Autodesk Inventor part; units mm, degrees
ref_plane "YZ Plane" through (0, 0, 0) normal (1, 0, 0) x (0, 1, 0)
ref_plane "XZ Plane" through (0, 0, 0) normal (0, 1, 0) x (-1, 0, 0)
ref_plane "XY Plane" through (0, 0, 0) normal (0, 0, 1) x (1, 0, 0)
sketch "Sketch1" plane through (0, 0, 0) normal (0, 1, 0) x (-1, 0, 0)
  arc A0 (7, 0) -> (-7, 0) centre (0, 0) ccw
  circle A1 centre (0, 0) radius 4
  line L0 (-7, 0) -> (-7, -83)
  line L1 (-7, -83) -> (7, -83)
  line L2 (7, -83) -> (7, 0)
  point P0 (0, -83)
  dimension "d0" = 14
  dimension "d1" = 8
  dimension "d2" = 83
  dimension "d3" = 14
  dimension "d4" = 83
  dimension "d5" = 0
extrude "Extrusion1" add sketch "Sketch1" along normal blind 20
sketch "Sketch2" plane through (7, 0, 0) normal (1, 0, 0) x (0, 0, -1)
  line L0 (0, 20) -> (83, 20)
  line L1 (83, 0) -> (83, 20)
  line L2 (83, 20) -> (81.9518, 0)
  line L3 (83, 20) -> (107.3414, 20) construction
  line L4 (83, 20) -> (83, 0)
  line L5 (83, 0) -> (81.9518, 0)
  line L6 (0, 0) -> (83, 0)
  dimension "d9" = 93
extrude "Extrusion2" cut sketch "Sketch2" against normal through all
sketch "Sketch3" plane through (7, 0, 0) normal (1, 0, 0) x (0, 0, -1)
  line L0 (-7, 6) -> (8, 6)
  line L1 (8, 6) -> (8, 14)
  line L2 (8, 14) -> (-7, 14)
  line L3 (-7, 14) -> (-7, 6)
  line L4 (-7, 6) -> (8, 14) construction
  line L5 (8, 6) -> (-7, 14) construction
  point P0 (0, 0)
  point P1 (0.5, 10)
  dimension "d12" = 10
  dimension "d13" = 15
  dimension "d14" = 8
  dimension "d15" = 7
extrude "Extrusion3" cut sketch "Sketch3" against normal through all
chamfer "Chamfer1" distance 0.5 angle 45 6 edges at (7, 0, -40.9759) (0, 0, 7) (-7, 0, -40.9759) (7, 20, -41.5) (0, 20, 7) (-7, 20, -41.5)
properties part number "Schneidstempel"
Source: CAD feature listing. Evaluate the final solid. Frame: model axes, mm. A direction names the side the tool comes from. Coordinates: 2 decimals unless noted, no trailing zeros. Order: outer loops, then holes, each group sorted by start corner. A loop starts at its lowest first (then second) coordinate and runs counter-clockwise, first axis right, second up. Notation, with made-up numbers: M -8,40 L 39,40 A28 ccw 39,58 Z; hole C 55,33.5 d1. An arc over 180 degrees is marked long. Write each question's results on one line, items separated by ' | '. Start each with the question number.
1) Line query: line 1 (X direction, y = 18.85, z = 0); line 2 (Y direction, x = 5.75, z = 1); line 3 (X direction, y = 3.75, z = -2.5). Output: solid intervals per line, ascending. Write a range as from..to.
2) Section query C-C (y = 12). Return the cut outline in (x, z).
3) Section query B-B (y = 1.75). Return the cut outline in (x, z), plus the area to 3 significant figures.
4) Access query for faces 4 (the face through (0.098, 10.14, -82.483)), 5 (the face through (2, 14, -4)). Directions: +Z, -Z, +X, -X, +Y, -Y. A direction counts if a zero-diameter tool reaches every point of the face in a straight line with its end or side. Return the directions, or none.
5) Contact query for flat-ended pins moving along their axis: pin 1 Ø1.5 at (x, y) = (-4.5, 14.5) entering from -Z; pin 2 Ø5 at (x, z) = (0, 0) entering from +Y; pin 3 Ø5 at (x, y) = (-5.5, 16) entering from +Z. Output: stop coordinate, or through.
6) Draft query along Z for faces 1 (the face through (-7, 10, -42)), 2 (the face through (0, 3, 7)), 3 (the face through (0.867, 16.958, 3.905)). Return one class per face: released by +Z, released by -Z, zero draft, split by the parting line, or undercut.
7) Section query D-D (y = 7.75). Return the cut outline in (x, z).
8) Section query A-A (x = 0). Return the cut outline in (y, z), plus the area to 3 significant figures.
Answers:
1) line 1: x = -7..-4, 4..7 | line 2: y = 0..6, 14..20 | line 3: x = -7..-3.12, 3.12..7
2) outline: M -7,-82.58 L 7,-82.58 L 7,-8 L -7,-8 Z
3) outline: M -7,-82.04 L 7,-82.04 L 7,0 A7 ccw -7,0 Z; hole C 0,0 d8 | area: 1,180 mm^2
4) face 4: -Z, +X, -X, -Y | face 5: +Z, +X, -X
5) pin 1: stops at z = -82.75 | pin 2: passes through | pin 3: stops at z = 6.32
6) face 1: zero draft | face 2: released by +Z | face 3: undercut
7) outline: M -7,-82.36 L 7,-82.36 L 7,-8 L -7,-8 Z
8) outline: M 0,-81.95 L 20,-83 L 20,-4 L 14,-4 L 14,-8 L 6,-8 L 6,-4 L 0,-4 Z; M 0,4 L 6,4 L 6,7 L 0.5,7 L 0,6.5 Z; M 14,4 L 20,4 L 20,6.5 L 19.5,7 L 14,7 Z | area: 1,570 mm^2
